Source: CAD feature listing. Evaluate the final solid. Frame: model axes, mm. Give positions to 0.01 mm unless a question says otherwise; leave off trailing zeros. Order: outer loops, then holes, each group sorted by start corner. A loop starts at its lowest first (then second) coordinate and runs counter-clockwise, first axis right, second up.
1) First-contact query: P1, Ø3, axis at y = -55.5, z = -2.5, coming from the +X side; P2, Ø1, axis at y = 14, z = -5, coming from the -X side; P3, Ø2, axis at y = -1.5, z = -5.5, coming from the -X side. Flat tips, straight axial feed; report the tip coordinate or a pass-through.
2) Material intervals for line 1 (Y direction, x = -36, z = -0.25); line 2 (Y direction, x = -28.5, z = -2.25); line 3 (X direction, y = -3, z = -3.75), sorted ascending.
3) Section A-A, the plane y = -2.5. Return loops of the section in (x, z).
4) Section B-B, the plane z = -5. Give the number of separate pieces and of enclosed holes in the cut face, plus the area to 3 significant figures.
```python
from build123d import *

# Parameters (mm, degrees)
CHAMFER1_SIZE                  = 2
SKETCH3_R                      = 4.1021
CUT_EXTRUDE2_DEPTH             = 7
SKETCH5_R                      = 6.54812
CUT_EXTRUDE3_DEPTH             = 7
SKETCH10_OUTSIDE_W             = 204.706
SKETCH10_OUTSIDE_H             = 204.706
CUT_EXTRUDELIGHTENSPIDER_DEPTH = 7


with BuildPart() as part:
    # Sketch1 → Revolve1 (revolve)
    with BuildSketch(Plane(origin=(0, 0, 0), x_dir=(0, 0, -1), z_dir=(1, 0, 0))):
        Polygon((2, 79), (6, 79), (6, 58.75), (6, 30.4), (0, 30.4), (0, 60.4), (0, 79), align=None)
    revolve(axis=Axis((0, 0, 42.402729345), (0, 0, -1)))

    # Chamfer1
    chamfer1_edges = [part.edges().sort_by_distance(p)[0] for p in [
        (0, -30.4, 0),
    ]]
    chamfer(chamfer1_edges, length=CHAMFER1_SIZE)

    # Sketch3 → Cut-Extrude2 (cut, through all)
    with BuildSketch(Plane.XY):
        with Locations((0, 69.85)):
            Circle(SKETCH3_R)
        with Locations((60.491874454, 34.925)):
            Circle(SKETCH3_R)
        with Locations((60.491874454, -34.925)):
            Circle(SKETCH3_R)
        with Locations((0, -69.85)):
            Circle(SKETCH3_R)
        with Locations((-60.491874454, -34.925)):
            Circle(SKETCH3_R)
        with Locations((-60.491874454, 34.925)):
            Circle(SKETCH3_R)
    extrude(amount=-CUT_EXTRUDE2_DEPTH, mode=Mode.SUBTRACT)

    # Sketch5 → Cut-Extrude3 (cut, through all)
    with BuildSketch(Plane.XY):
        with Locations((0, 47.6)):
            Circle(SKETCH5_R)
        with Locations((47.6, 0)):
            Circle(SKETCH5_R)
        with Locations((0, -47.6)):
            Circle(SKETCH5_R)
        with Locations((-47.6, 0)):
            Circle(SKETCH5_R)
    extrude(amount=-CUT_EXTRUDE3_DEPTH, mode=Mode.SUBTRACT)

    # Sketch10 outside → Cut-ExtrudeLightenSpider (cut, through all)
    with BuildSketch(Plane.XY):
        Rectangle(SKETCH10_OUTSIDE_W, SKETCH10_OUTSIDE_H)
        with BuildLine():
            Line((-10.026404015, 65.791524605), (-15.612126757, 57.594828522))
            ThreePointArc((-15.612126757, 57.594828522), (-22.370889622, 50.893885768), (-31.144282145, 47.204564302))
            Line((-31.144282145, 47.204564302), (-52.913637786, 42.643181716))
            ThreePointArc((-52.913637786, 42.643181716), (-54.833820547, 42.555428057), (-56.683216005, 43.079392731))
            ThreePointArc((-56.683216005, 43.079392731), (-67.808926528, 40.165300464), (-66.985857737, 28.693773706))
            ThreePointArc((-66.985857737, 28.693773706), (-66.607453407, 28.208181309), (-66.336137509, 27.655571594))
            Line((-66.336137509, 27.655571594), (-58.910187887, 7.538148679))
            ThreePointArc((-58.910187887, 7.538148679), (-58.726829376, 6.382845568), (-58.999242441, 5.245244256))
            ThreePointArc((-58.999242441, 5.245244256), (-60.103553413, -1.056630301), (-57.957357907, -7.083816253))
            ThreePointArc((-57.957357907, -7.083816253), (-57.456302519, -8.408967742), (-57.619209975, -9.816285805))
            Line((-57.619209975, -9.816285805), (-63.372036652, -25.401100289))
            ThreePointArc((-63.372036652, -25.401100289), (-63.921102493, -26.329038035), (-64.762782095, -27.002920227))
            ThreePointArc((-64.762782095, -27.002920227), (-68.5334328, -38.966452632), (-56.683216005, -43.079392731))
            ThreePointArc((-56.683216005, -43.079392731), (-54.833820547, -42.555428057), (-52.913637786, -42.643181716))
            Line((-52.913637786, -42.643181716), (-31.144282145, -47.204564302))
            ThreePointArc((-31.144282145, -47.204564302), (-22.370889622, -50.893885768), (-15.612126757, -57.594828522))
            Line((-15.612126757, -57.594828522), (-10.026404015, -65.791524605))
            ThreePointArc((-10.026404015, -65.791524605), (-9.212368611, -67.53283127), (-8.990756336, -69.442200417))
            ThreePointArc((-8.990756336, -69.442200417), (0, -78.85), (8.990756336, -69.442200417))
            ThreePointArc((8.990756336, -69.442200417), (9.212368611, -67.53283127), (10.026404015, -65.791524605))
            Line((10.026404015, -65.791524605), (15.612126757, -57.594828522))
            ThreePointArc((15.612126757, -57.594828522), (22.370889622, -50.893885768), (31.144282145, -47.204564302))
            Line((31.144282145, -47.204564302), (52.913637786, -42.643181716))
            ThreePointArc((52.913637786, -42.643181716), (54.833820547, -42.555428057), (56.683216005, -43.079392731))
            ThreePointArc((56.683216005, -43.079392731), (67.808926528, -40.165300464), (66.985857737, -28.693773706))
            ThreePointArc((66.985857737, -28.693773706), (66.607453407, -28.208181309), (66.336137509, -27.655571594))
            Line((66.336137509, -27.655571594), (58.910187887, -7.538148679))
            ThreePointArc((58.910187887, -7.538148679), (58.726829376, -6.382845568), (58.999242441, -5.245244256))
            ThreePointArc((58.999242441, -5.245244256), (60.103553413, 1.056630301), (57.957357907, 7.083816253))
            ThreePointArc((57.957357907, 7.083816253), (57.456302519, 8.408967742), (57.619209975, 9.816285805))
            Line((57.619209975, 9.816285805), (63.004017141, 24.404109395))
            ThreePointArc((63.004017141, 24.404109395), (63.949907854, 26.077457327), (65.376417653, 27.365817654))
            ThreePointArc((65.376417653, 27.365817654), (68.367056511, 39.2817772), (56.683216005, 43.079392731))
            ThreePointArc((56.683216005, 43.079392731), (54.833820547, 42.555428057), (52.913637786, 42.643181716))
            Line((52.913637786, 42.643181716), (31.144282145, 47.204564302))
            ThreePointArc((31.144282145, 47.204564302), (22.370889622, 50.893885768), (15.612126757, 57.594828522))
            Line((15.612126757, 57.594828522), (10.026404015, 65.791524605))
            ThreePointArc((10.026404015, 65.791524605), (9.212368611, 67.53283127), (8.990756336, 69.442200417))
            ThreePointArc((8.990756336, 69.442200417), (0, 78.85), (-8.990756336, 69.442200417))
            ThreePointArc((-8.990756336, 69.442200417), (-9.212368611, 67.53283127), (-10.026404015, 65.791524605))
        make_face(mode=Mode.SUBTRACT)
        with BuildLine():
            Line((-38.171337153, -19.163288775), (-30.989327096, -29.702435886))
            ThreePointArc((-30.989327096, -29.702435886), (-30.974904193, -33.059883994), (-34.083658328, -34.328077016))
            Line((-34.083658328, -34.328077016), (-46.782801613, -31.667196649))
            ThreePointArc((-46.782801613, -31.667196649), (-50.132508933, -29.193901063), (-50.448043328, -25.042013753))
            Line((-50.448043328, -25.042013753), (-48.758289676, -20.464351561))
            ThreePointArc((-48.758289676, -20.464351561), (-43.861379511, -16.586899466), (-38.171337153, -19.163288775))
        make_face()
        with BuildLine():
            Line((-48.823135839, 36.348261242), (-29.399536951, 40.418132082))
            ThreePointArc((-29.399536951, 40.418132082), (-28.363285572, 39.995401074), (-28.368093206, 38.876251705))
            Line((-28.368093206, 38.876251705), (-41.341857561, 19.838070188))
            ThreePointArc((-41.341857561, 19.838070188), (-44.186878741, 18.549875534), (-46.635333823, 20.488601581))
            Line((-46.635333823, 20.488601581), (-51.022280868, 32.373151504))
            ThreePointArc((-51.022280868, 32.373151504), (-50.832960232, 34.86428389), (-48.823135839, 36.348261242))
        make_face()
        with BuildLine():
            Line((46.635333823, -20.488601581), (51.022280868, -32.373151504))
            ThreePointArc((51.022280868, -32.373151504), (50.832960232, -34.86428389), (48.823135839, -36.348261242))
            Line((48.823135839, -36.348261242), (29.399536951, -40.418132082))
            ThreePointArc((29.399536951, -40.418132082), (28.363285572, -39.995401074), (28.368093206, -38.876251705))
            Line((28.368093206, -38.876251705), (41.341857561, -19.838070188))
            ThreePointArc((41.341857561, -19.838070188), (44.186878741, -18.549875534), (46.635333823, -20.488601581))
        make_face()
        with BuildLine():
            Line((34.083658328, 34.328077016), (46.782801613, 31.667196649))
            ThreePointArc((46.782801613, 31.667196649), (50.132508933, 29.193901063), (50.448043328, 25.042013753))
            Line((50.448043328, 25.042013753), (48.758289676, 20.464351561))
            ThreePointArc((48.758289676, 20.464351561), (43.861379511, 16.586899466), (38.171337153, 19.163288775))
            Line((38.171337153, 19.163288775), (30.989327096, 29.702435886))
            ThreePointArc((30.989327096, 29.702435886), (30.974904193, 33.059883994), (34.083658328, 34.328077016))
        make_face()
        with BuildLine():
            Line((-15.821171438, 41.306107758), (-35.834530202, 11.937765116))
            ThreePointArc((-35.834530202, 11.937765116), (-36.35519159, 10.21012461), (-35.790664462, 8.496316242))
            ThreePointArc((-35.790664462, 8.496316242), (-33.058727226, 0.446297704), (-35.291848474, -7.756107371))
            ThreePointArc((-35.291848474, -7.756107371), (-35.75327476, -9.409318188), (-35.232852266, -11.044916137))
            Line((-35.232852266, -11.044916137), (-18.616205445, -35.42879808))
            ThreePointArc((-18.616205445, -35.42879808), (-13.39288563, -38.802460256), (-7.331267504, -37.416295746))
            ThreePointArc((-7.331267504, -37.416295746), (2.539818576, -35.311605592), (10.767731208, -41.157075185))
            ThreePointArc((10.767731208, -41.157075185), (13.253641017, -42.61539929), (15.821171438, -41.306107758))
            Line((15.821171438, -41.306107758), (35.834530202, -11.937765117))
            ThreePointArc((35.834530202, -11.937765117), (36.35519159, -10.21012461), (35.790664462, -8.496316242))
            ThreePointArc((35.790664462, -8.496316242), (33.058727226, -0.446297704), (35.291848474, 7.756107371))
            ThreePointArc((35.291848474, 7.756107371), (35.75327476, 9.409318188), (35.232852266, 11.044916137))
            Line((35.232852266, 11.044916137), (18.616205445, 35.42879808))
            ThreePointArc((18.616205445, 35.42879808), (13.39288563, 38.802460256), (7.331267504, 37.416295746))
            ThreePointArc((7.331267504, 37.416295746), (-2.539818576, 35.311605592), (-10.767731208, 41.157075185))
            ThreePointArc((-10.767731208, 41.157075185), (-13.253641017, 42.61539929), (-15.821171438, 41.306107758))
        make_face()
    extrude(amount=-CUT_EXTRUDELIGHTENSPIDER_DEPTH, mode=Mode.SUBTRACT)


solid = part.part
```
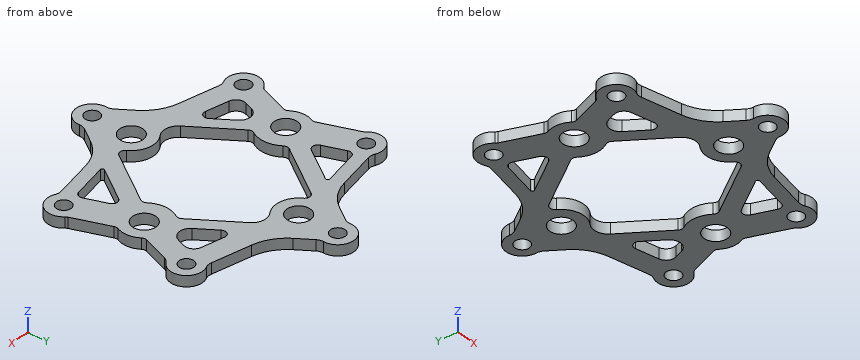
From the geometry:
1. P1: stops at x = 18.59
1. P2: stops at x = -61.48
1. P3: stops at x = -60.14
2. line 1: y = -46.19 to -33.93, -22.35 to 8.83, 11.66 to 27.68, 39.04 to 46.19
2. line 2: y = -47.91 to -20.92, 22.7 to 38.68, 40.16 to 47.91
2. line 3: x = -59.78 to -53.42, -41.78 to -33.36, 33.36 to 41.78, 53.42 to 59.78
3. outline: (-59.9, -6) - (-53.65, -6) - (-53.65, 0) - (-59.9, 0) - close; (-41.55, -6) - (-33.27, -6) - (-33.27, 0) - (-41.55, 0) - close; (33.27, -6) - (41.55, -6) - (41.55, 0) - (33.27, 0) - close; (53.65, -6) - (59.9, -6) - (59.9, 0) - (53.65, 0) - close
4. separate pieces: 1
4. enclosed holes: 15
4. area: 7,080 mm2
